Design review of the part built by this model. Coordinates are the model's own, in mm. Face numbers are marked on the shaded views. A direction names the side the tool comes from. Coordinates: 2 decimals unless noted, no trailing zeros. Write each loop counter-clockwise with the first axis right and the second up, starting at its lowest first coordinate (ties: lowest second). Pieces come first, ordered by that corner, then holes.
Q1. Take a section at A-A (z = 7.5). Give the boundary of the cut face in (x, y).
Q2. Insertion check: pin 1 (10 mm diameter, centred on x = 23.5, z = 9, fed in from -Y); pin 2 (12 mm diameter, centred on x = -2, z = 24, fed in from +Y); pin 3 (1 mm diameter, centred on y = -5.5, z = 10.5, fed in from +X); pin 4 (20 mm diameter, centred on x = -18, z = 26, fed in from -Y). Each pin has a flat end and moves straight along its axis. Give the tip position at first contact, or say it passes through.
Q3. For probe 1 along X at (y, z) = (8.5, 15); probe 2 along Y at (x, z) = (21.5, 8.5); probe 3 along Z at (x, y) = (21, -2), list the stretches that pass through material, from the lowest coordinate up.
Q4. Machinability: for the marked faces 4, 5 and 6, which of the approach directions +Z, -Z, +X, -X, +Y, -Y give a long, thin tool a straight path to every point of the face, cutting with its end or side? Answer none if there is none.
Q5. Take a section at D-D (y = -8.5). Give the boundary of the cut face in (x, z), and give its area (3 significant figures).
Q6. Take a section at B-B (y = 14). Give the boundary of the cut face in (x, z).
Q7. Mouldability with a two-part tool opening along X and no side actions: class the marked faces 1, 2 and 3 as pulls with the +X half, pulls with the -X half, needs draft (parallel to the pull), parting line crosses it, or undercut.
Q8. Take a section at C-C (x = -15.5). Give the boundary of the cut face in (y, z).
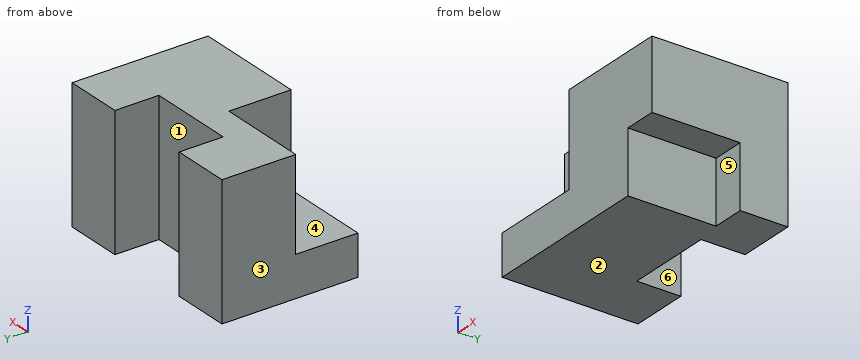
```python
from build123d import *

# Parameters (mm, degrees)
F1_DEPTH = 35.9918
F2_W     = 24.003
F2_H     = 16.9418
F3_DEPTH = 8.9916
F4_W     = 24.9682
F4_H     = 24.9428
F5_DEPTH = 16.9418


with BuildPart() as f1:
    # F0 (on Top) → F1 (new body)
    with BuildSketch(Plane.XY):
        Polygon((28.0035, -18.5039), (28.0035, 18.5039), (12.0015, 18.5039), (12.0015, 6.5151), (-12.0015, 6.5151), (-12.0015, 18.5039), (-28.0035, 18.5039), (-28.0035, -18.5039), align=None)
    extrude(amount=F1_DEPTH)

    # F2 (on face) → F3 (cut)
    with BuildSketch(Plane.YZ.offset(28.0035)):
        with Locations((-6.5024, 8.4709)):
            Rectangle(F2_W, F2_H)
    extrude(amount=-F3_DEPTH, mode=Mode.SUBTRACT)

    # F4 (on face) → F5 (cut)
    with BuildSketch(Plane.XZ.offset(18.5039)):
        with Locations((-15.5194, 23.5204)):
            Rectangle(F4_W, F4_H)
    extrude(amount=-F5_DEPTH, mode=Mode.SUBTRACT)


solid = f1.part
```
Response:
1. outline: (-28, -18.5) - (19.01, -18.5) - (19.01, 5.5) - (28, 5.5) - (28, 18.5) - (12, 18.5) - (12, 6.52) - (-12, 6.52) - (-12, 18.5) - (-28, 18.5) - close
2. pin 1: stops at y = -18.5
2. pin 2: stops at y = 6.52
2. pin 3: stops at x = 19.01
2. pin 4: stops at y = -1.56
3. probe 1: x = -28 to -12, 12 to 28
3. probe 2: y = 5.5 to 18.5
3. probe 3: z = 16.94 to 35.99
4. face 4: +Z, -X, -Y
4. face 5: -Z, +X, -Y
4. face 6: +Z, -Z, +Y
5. outline: (-28, 0) - (19.01, 0) - (19.01, 16.94) - (28, 16.94) - (28, 35.99) - (-3.04, 35.99) - (-3.04, 11.05) - (-28, 11.05) - close
5. area: 1,240 mm2
6. outline: (-28, 0) - (-12, 0) - (-12, 35.99) - (-28, 35.99) - close; (12, 0) - (28, 0) - (28, 35.99) - (12, 35.99) - close
7. face 1: undercut
7. face 2: needs draft
7. face 3: pulls with the -X half
8. outline: (-18.5, 0) - (18.5, 0) - (18.5, 35.99) - (-1.56, 35.99) - (-1.56, 11.05) - (-18.5, 11.05) - close
